Answer from the drawing. Dimensions are ordinates in mm from the lowest x, y and z of the part. Round coordinates to 2 decimals unless told otherwise and drop trailing zeros. Write each loop counter-clockwise with the first axis right and the second up, starting at its lowest first coordinate (ties: lowest second). Pieces come first, ordered by that corner, then holes. Notation, with made-up numbers: M 53.25,33 L 110.25,33 A10 cw 110.25,39 Z; hole C -5.5,2.25 d1. An arc over 180 degrees is marked long. Answer as CSV lines item,"result". Start each with the question number.
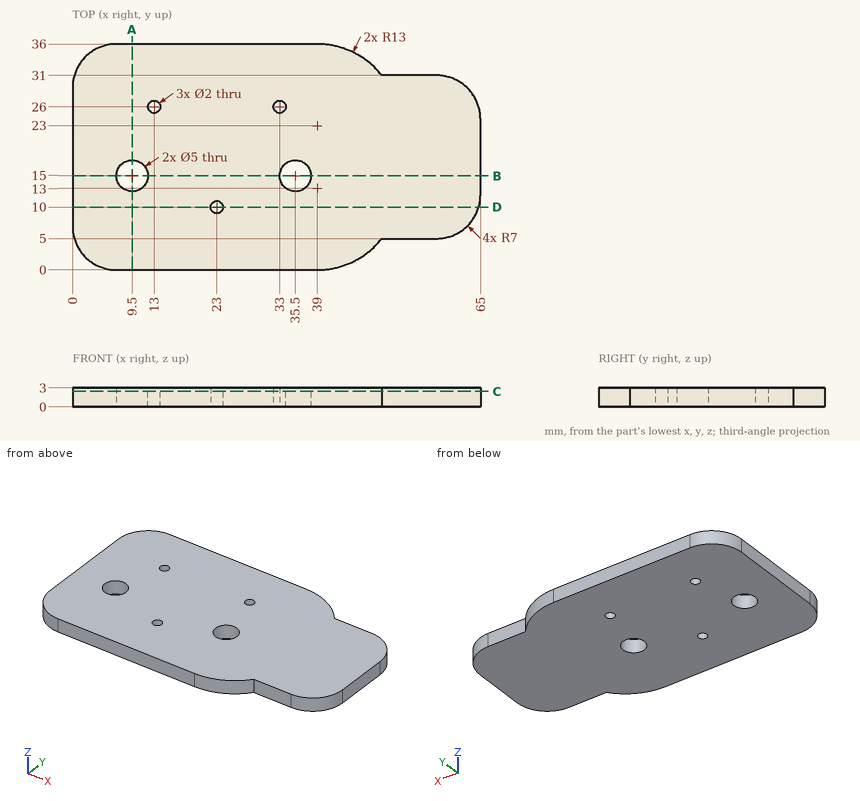
Q1. Find section D-D (y = 10). Determine the outline of the cut face in (x, z).
Q2. Find section A-A (x = 9.5). Determine the outline of the cut face in (y, z).
Q3. Each of these flat-tipped pins is pushed along its axis until it touches: P1, Ø1.5, axis at x = 52.5, z = 2, coming from the +Y side; P2, Ø1.8, axis at x = 23, y = 10, coming from the -Z side. Where does it stop, or does it pass through?
Q4. Straight lines are drawn through the part: L1, parallel to X at y = 26, z = 2.55; L2, parallel to Y at x = 35.5, z = 1.2; L3, parallel to X at y = 13.5, z = 1.2. For each, find the intervals that lie inside material, in ascending order.
Q5. Find section B-B (y = 15). Determine the outline of the cut face in (x, z), plus the area to 3 significant figures.
Q6. Find section C-C (z = 2.45). Determine the outline of the cut face in (x, y).
Reported:
1,outline,"M 0,0 L 22,0 L 22,3 L 0,3 Z; M 24,0 L 64.71,0 L 64.71,3 L 24,3 Z"
2,outline,"M 0,0 L 12.5,0 L 12.5,3 L 0,3 Z; M 17.5,0 L 36,0 L 36,3 L 17.5,3 Z"
3,P1,"stops at y = 31"
3,P2,"passes through"
4,L1,"x = 0 to 12, 14 to 32, 34 to 64.71"
4,L2,"y = 0 to 12.5, 17.5 to 36"
4,L3,"x = 0 to 7.5, 11.5 to 33.5, 37.5 to 65"
5,outline,"M 0,0 L 7,0 L 7,3 L 0,3 Z; M 12,0 L 33,0 L 33,3 L 12,3 Z; M 38,0 L 65,0 L 65,3 L 38,3 Z"
5,area,"165 mm2"
6,outline,"M 0,7 A7 ccw 7,0 L 39,0 A13 ccw 49.25,5 L 58,5 A7 ccw 65,12 L 65,24 A7 ccw 58,31 L 49.25,31 A13 ccw 39,36 L 7,36 A7 ccw 0,29 Z; hole C 9.5,15 d5; hole C 13,26 d2; hole C 23,10 d2; hole C 33,26 d2; hole C 35.5,15 d5"
